from build123d import *

# Parameters (mm, degrees)
SKETCH1_R           = 14
BOSS_EXTRUDE1_DEPTH = 34
SKETCH2_R           = 8.5
BOSS_EXTRUDE2_DEPTH = 2
SKETCH3_R           = 3
BOSS_EXTRUDE3_DEPTH = 17
FILLET1_R           = 0.5
SKETCH5_R           = 14
BOSS_EXTRUDE4_DEPTH = 26
CHAMFER1_SIZE       = 2
CHAMFER1_SIZE2      = 1.154700538
SKETCH6_R           = 6
CUT_EXTRUDE1_DEPTH  = 57


with BuildPart() as part:
    # Sketch1 → Boss-Extrude1 (new body)
    with BuildSketch(Plane(origin=(0, 0, 0), x_dir=(1, 0, 0), z_dir=(0, 1, 0))):
        Circle(SKETCH1_R)
    extrude(amount=BOSS_EXTRUDE1_DEPTH)

    # Sketch2 → Boss-Extrude2 (add)
    with BuildSketch(Plane(origin=(0, 34, 0), x_dir=(1, 0, 0), z_dir=(0, 1, 0))):
        Circle(SKETCH2_R)
    extrude(amount=BOSS_EXTRUDE2_DEPTH)

    # Sketch3 → Boss-Extrude3 (add)
    with BuildSketch(Plane(origin=(0, 36, 0), x_dir=(1, 0, 0), z_dir=(0, 1, 0))):
        Circle(SKETCH3_R)
    extrude(amount=BOSS_EXTRUDE3_DEPTH)

    # Fillet1
    fillet1_edges = [part.edges().sort_by_distance(p)[0] for p in [
        (-14, 0, 0),
        (-14, 34, 0),
    ]]
    fillet(fillet1_edges, radius=FILLET1_R)

    # Sketch5 → Boss-Extrude4 (add)
    with BuildSketch(Plane.XZ):
        Circle(SKETCH5_R)
    extrude(amount=BOSS_EXTRUDE4_DEPTH)

    # Chamfer1
    chamfer1_edges = [part.edges().sort_by_distance(p)[0] for p in [
        (-14, -26, 0),
    ]]
    chamfer1_side = [part.faces().sort_by_distance(p)[0] for p in [
        (-14, -13, 0),
    ]]
    chamfer(chamfer1_edges, length=CHAMFER1_SIZE, length2=CHAMFER1_SIZE2, reference=chamfer1_side[0])

    # Sketch6 → Cut-Extrude1 (cut)
    with BuildSketch(Plane.XZ.offset(26)):
        Circle(SKETCH6_R)
    extrude(amount=-CUT_EXTRUDE1_DEPTH, mode=Mode.SUBTRACT)


solid = part.part
The model under review builds one solid part; all positions refer to its coordinate system, in mm. A direction names the side the tool comes from. Round coordinates to 2 decimals unless told otherwise and drop trailing zeros. Write each loop counter-clockwise with the first axis right and the second up, starting at its lowest first coordinate (ties: lowest second). Pieces come first, ordered by that corner, then holes. Notation, with made-up numbers: M -30.5,15 L 17.5,15 A18 ccw 17.5,31 Z; hole C 61,-3 d1. An arc over 180 degrees is marked long. Use a Markdown table: item, result. Add a question column.
Q1. Machinability: for faces 4 (the face through (-6, 2, 0)), 5 (the face through (-3, 44, 0)), 6 (the face through (0, 53, 0)), which of the approach directions +Z, -Z, +X, -X, +Y, -Y give a long, thin tool a straight path to every point of the face, cutting with its end or side? Answer none if there is none.
Q2. We need section A-A, the plane x = 0. State the section outline as (y, z) points, plus the area to 3 significant figures.
Q3. Insertion check: pin 1 (3.5 mm diameter, centred on x = -3, z = -1.5, fed in from -Y); pin 2 (8 mm diameter, centred on y = 2, z = 10.5, fed in from +X); pin 3 (6 mm diameter, centred on x = -6.5, y = 35, fed in from -Z). Each pin has a flat end and moves straight along its axis. Give the tip position at first contact, or say it passes through.
Q4. We need section B-B, the plane z = 0. State the section outline as (x, y) points.
Q5. We need section C-C, the plane y = 25. State the section outline as (x, z) points.
Q6. To check wall thickness, follow line 1 (Z direction, x = 0, y = -4); line 2 (Y direction, x = 9.5, z = -0.75); line 3 (Z direction, x = -2.25, y = -18). State the ranges of each line that lie inside material, in increasing order.
Q7. The part is to be moulded in two halves that separate along Z. For faces 1 (the face through (0, 31, 0)), 2 (the face through (9, 34, 0)), 3 (the face through (4.57, 34.986, -7.167)), say which applies: pulls with the +Z half, pulls with the -Z half, needs draft (parallel to the pull), parting line crosses it, or undercut.
Findings below:
| question | item | result |
|---|---|---|
| 1 | face 4 | -Y |
| 1 | face 5 | +Y |
| 1 | face 6 | +Z, -Z, +X, -X, +Y |
| 2 | outline | M -26,-12.85 L -24,-14 L 0,-14 L 0,-13.5 A0.5 ccw 0.5,-14 L 33.5,-14 A0.5 ccw 34,-13.5 L 34,-8.5 L 36,-8.5 L 36,-3 L 53,-3 L 53,3 L 36,3 L 36,8.5 L 34,8.5 L 34,13.5 A0.5 ccw 33.5,14 L 0.5,14 A0.5 ccw 0,13.5 L 0,14 L -24,14 L -26,12.85 L -26,6 L 31,6 L 31,-6 L -26,-6 Z |
| 2 | area | 1,130 mm² |
| 3 | pin 1 | stops at y = 31 |
| 3 | pin 2 | stops at x = 12.4 |
| 3 | pin 3 | stops at z = -13.45 |
| 4 | outline | M -14,-24 L -12.85,-26 L -6,-26 L -6,31 L 6,31 L 6,-26 L 12.85,-26 L 14,-24 L 14,0 L 13.5,0 A0.5 ccw 14,0.5 L 14,33.5 A0.5 ccw 13.5,34 L 8.5,34 L 8.5,36 L 3,36 L 3,53 L -3,53 L -3,36 L -8.5,36 L -8.5,34 L -13.5,34 A0.5 ccw -14,33.5 L -14,0.5 A0.5 ccw -13.5,0 L -14,0 Z |
| 5 | outline | C 0,0 d28; hole C 0,0 d12 |
| 6 | line 1 | z = -14 to -6, 6 to 14 |
| 6 | line 2 | y = -26 to 34 |
| 6 | line 3 | z = -13.82 to -5.56, 5.56 to 13.82 |
| 7 | face 1 | undercut |
| 7 | face 2 | needs draft |
| 7 | face 3 | parting line crosses it |
